The model under review builds one solid part; all positions refer to its coordinate system, in mm. A direction names the side the tool comes from. Round coordinates to 2 decimals unless told otherwise and drop trailing zeros. Write each loop counter-clockwise with the first axis right and the second up, starting at its lowest first coordinate (ties: lowest second). Pieces come first, ordered by that corner, then holes. Notation, with made-up numbers: (40.5, -35) -> (84.5, -35) arc R15 ccw to (84.5, -15) -> close; hole circle Ø5 at (70, -15.75). An arc over 180 degrees is marked (long way). Answer in a Markdown table with one row per item. Add a question column.
```python
from build123d import *

# Parameters (mm, degrees)
BOX005_W                    = 10
BOX005_H                    = 13
BOX005_DEPTH                = 4
BOX004_W                    = 3
BOX004_H                    = 31
BOX004_DEPTH                = 14
BOX003_W                    = 2
BOX003_H                    = 33
BOX003_DEPTH                = 11.2
BOX002_W                    = 9
BOX002_H                    = 35
BOX002_DEPTH                = 26
EXTRUDE_DEPTH               = 5
EXTRUDE001_DEPTH            = 5
THICKNESS_T                 = 1
BOX_W                       = 12
BOX_H                       = 31
BOX_DEPTH                   = 15
BOX001_W                    = 13
BOX001_H                    = 34
BOX001_DEPTH                = 14
CYLINDER001_W               = 48
CYLINDER001_H               = 15
CYLINDER001_ANGLE           = 60
CYLINDER001_PLACEMENT_ANGLE = 60
CYLINDER_W                  = 51
CYLINDER_H                  = 15
CYLINDER_ANGLE              = 60
CYLINDER_PLACEMENT_ANGLE    = 60


with BuildPart() as servo_wall_cutaway:
    # Box005 → Box005 (new body)
    with BuildSketch(Plane(origin=(-6, 19.5, 10), x_dir=(1, 0, 0), z_dir=(0, 0, 1))):
        with Locations((5, 6.5)):
            Rectangle(BOX005_W, BOX005_H)
    extrude(amount=BOX005_DEPTH)


with BuildPart() as slot_wall_cutout2:
    # Box004 → Box004 (new body)
    with BuildSketch(Plane(origin=(-1, 7, 14), x_dir=(1, 0, 0), z_dir=(0, 0, 1))):
        with Locations((1.5, 15.5)):
            Rectangle(BOX004_W, BOX004_H)
    extrude(amount=BOX004_DEPTH)


with BuildPart() as slot_wall_cutout1:
    # Box003 → Box003 (new body)
    with BuildSketch(Plane(origin=(-0.5, 6, 20), x_dir=(1, 0, 0), z_dir=(0, 0, 1))):
        with Locations((1, 16.5)):
            Rectangle(BOX003_W, BOX003_H)
    extrude(amount=BOX003_DEPTH)


with BuildPart() as wall_slot_finished:
    # Box002 → Box002 (new body)
    with BuildSketch(Plane(origin=(-3, 5, 0), x_dir=(1, 0, 0), z_dir=(0, 0, 1))):
        with Locations((4.5, 17.5)):
            Rectangle(BOX002_W, BOX002_H)
    extrude(amount=BOX002_DEPTH)

    # Cut003: cut slot wall cutout1
    add(slot_wall_cutout1.part, mode=Mode.SUBTRACT)

    # Cut004: cut slot wall cutout2
    add(slot_wall_cutout2.part, mode=Mode.SUBTRACT)


with BuildPart() as wall_slot_finished_1:
    # Cut004 placement: moved
    add(wall_slot_finished.part.moved(Location((-3.3, -4.4, 0))))


with BuildPart() as extrude_body:
    with BuildSketch(Plane(origin=(8.5, 45, 6), x_dir=(1, 0, 0), z_dir=(0, 1, 0))):
        with BuildLine():
            Line((5, 4), (-5, 4))
            Line((-5, 4), (-5, -3.142136))
            ThreePointArc((-5, -3.142136), (-2.53653, -3.783978), (0, -4))
            ThreePointArc((0, -4), (2.53653, -3.783978), (5, -3.142136))
            Line((5, -3.142136), (5, 4))
        make_face()
    extrude(amount=EXTRUDE_DEPTH)


with BuildPart() as extrude001:
    with BuildSketch(Plane(origin=(8.5, 45, 6), x_dir=(1, 0, 0), z_dir=(0, 1, 0))):
        with BuildLine():
            Line((5, 4), (-5, 4))
            Line((-5, 4), (-5, -3.142136))
            ThreePointArc((-5, -3.142136), (-2.53653, -3.783978), (0, -4))
            ThreePointArc((0, -4), (2.53653, -3.783978), (5, -3.142136))
            Line((5, -3.142136), (5, 4))
        make_face()
    extrude(amount=EXTRUDE001_DEPTH)


with BuildPart() as bolt_bottle_side_opening:
    # Thickness base: copy of Extrude body
    add(extrude_body.part)

    # Thickness
    thickness_openings = [bolt_bottle_side_opening.faces().sort_by_distance(p)[0] for p in [
        (8.5, 50, 5.862901),
    ]]
    offset(amount=THICKNESS_T, openings=thickness_openings)

    # Fusion: union Extrude body, Extrude001
    add(extrude_body.part)
    add(extrude001.part)


with BuildPart() as bolt_bottle_side_opening_1:
    # Fusion placement: moved
    add(bolt_bottle_side_opening.part.moved(Location((0, -7, 1))))


with BuildPart() as pullbay:
    # Box → Box (new body)
    with BuildSketch(Plane(origin=(2.5, 7, 2), x_dir=(1, 0, 0), z_dir=(0, 0, 1))):
        with Locations((6, 15.5)):
            Rectangle(BOX_W, BOX_H)
    extrude(amount=BOX_DEPTH)


with BuildPart() as cut_bay_from_case:
    # Box001 → Box001 (new body)
    with BuildSketch(Plane(origin=(2, 6, 0), x_dir=(1, 0, 0), z_dir=(0, 0, 1))):
        with Locations((6.5, 17)):
            Rectangle(BOX001_W, BOX001_H)
    extrude(amount=BOX001_DEPTH)

    # Cut001: cut pullBay
    add(pullbay.part, mode=Mode.SUBTRACT)


with BuildPart() as bottle_wall001:
    # Cylinder001 → Cylinder001 (revolve)
    with BuildSketch(Plane.XZ):
        with Locations((24, 7.5)):
            Rectangle(CYLINDER001_W, CYLINDER001_H)
    revolve(axis=Axis((0, 0, 0), (0, 0, 1)), revolution_arc=CYLINDER001_ANGLE)


with BuildPart() as bottle_wall001_1:
    # Cylinder001 placement: moved
    add(bottle_wall001.part.moved(Location((8.5, -7, 0))).rotate(Axis((8.5, -7, 0), (0, 0, 1)), CYLINDER001_PLACEMENT_ANGLE))


with BuildPart() as cut005:
    # Cylinder → Cylinder (revolve)
    with BuildSketch(Plane.XZ):
        with Locations((25.5, 7.5)):
            Rectangle(CYLINDER_W, CYLINDER_H)
    revolve(axis=Axis((0, 0, 0), (0, 0, 1)), revolution_arc=CYLINDER_ANGLE)


with BuildPart() as cut005_1:
    # Cylinder placement: moved
    add(cut005.part.moved(Location((8.5, -7, 0))).rotate(Axis((8.5, -7, 0), (0, 0, 1)), CYLINDER_PLACEMENT_ANGLE))

    # Cut: cut bottle_wall001
    add(bottle_wall001_1.part, mode=Mode.SUBTRACT)


with BuildPart() as cut005_2:
    # Cut placement: moved
    add(cut005_1.part.moved(Location((0, -2, 0))))

    # Fusion001: union cut bay from case
    add(cut_bay_from_case.part)

    # Cut002: cut bolt_bottle_side_opening
    add(bolt_bottle_side_opening_1.part, mode=Mode.SUBTRACT)

    # Fusion002: union wall slot finished
    add(wall_slot_finished_1.part)

    # Cut005: cut servo wall cutaway
    add(servo_wall_cutaway.part, mode=Mode.SUBTRACT)


solid = cut005_2.part
```
1. Add section D-D on y = 14. Write out the cut boundary in (x, z), plus the area to 3 significant figures.
2. Insertion check: pin 1 Ø12 at (x, z) = (-2.5, 9.5) entering from +Y; pin 2 Ø8 at (x, y) = (10, 25.5) entering from +Z; pin 3 Ø4 at (x, z) = (8, 15.5) entering from -Y. Each pin has a flat end and moves straight along its axis. Give the tip position at first contact, or say it passes through.
3. Add section C-C on z = 7.75. Write out the cut boundary in (x, y), plus the area to 3 significant figures.
4. Add section A-A on y = 28. Write out the cut boundary in (x, z).
5. Tool access review of faces 4 (the flat face through (2, 37, 7)), 5 (the flat face through (-1.3, 18, 20)), 6 (the flat face through (-2, 0.6, 13)), 7 (the flat face through (2.5, 38, 8)): name each direction out of +Z, -Z, +X, -X, +Y, -Y from which nothing blocks a thin tool from reaching the whole face with its end or side.
6. Mouldability with a two-part tool opening along Z and no side actions: class faces 1 (the flat face through (14.7, 23.8, 14)), 2 (the flat face through (-6, 26, 12)), 3 (the flat face through (-4.3, 18, 20)) as pulls with the +Z half, pulls with the -Z half, needs draft (parallel to the pull), parting line crosses it, or undercut.
7. Add section B-B on x = -3. Write out the cut boundary in (y, z), plus the area to 3 significant figures.
8. For L1, parallel to Y at x = -4, z = 22; L2, parallel to X at y = 27, z = 10.75; L3, parallel to X at y = 7.5, z = 8.5, list the stretches that pass through material, from the lowest coordinate up.
Filled in:
| question | item | result |
|---|---|---|
| 1 | outline | (-6.3, 0) -> (15, 0) -> (15, 14) -> (14.5, 14) -> (14.5, 2) -> (2.7, 2) -> (2.7, 26) -> (-1.3, 26) -> (-1.3, 14) -> (-4.3, 14) -> (-4.3, 26) -> (-6.3, 26) -> close |
| 1 | area | 229 mm² |
| 2 | pin 1 | y = 41.73 |
| 2 | pin 2 | z = 2 |
| 2 | pin 3 | y = 6 |
| 3 | outline | (-17, 35.17) -> (-15.5, 32.57) arc R48 cw to (2, 38.56) -> (2, 35.6) -> (-6.3, 35.6) -> (-6.3, 0.6) -> (2.7, 0.6) -> (2.7, 6) -> (15, 6) -> (15, 38.56) arc R48 cw to (32.5, 32.57) -> (34, 35.17) arc R51 ccw to (14.5, 41.65) -> (14.5, 7) -> (2.7, 7) -> (2.7, 35.6) -> (2.5, 35.6) -> (2.5, 41.65) arc R51 ccw to start |
| 3 | area | 464 mm² |
| 4 | outline | (-6.3, 0) -> (15, 0) -> (15, 14) -> (14.5, 14) -> (14.5, 2) -> (2.7, 2) -> (2.7, 10) -> (-6, 10) -> (-6, 14) -> (-4.3, 14) -> (-4.3, 26) -> (-6.3, 26) -> close; (-1.3, 14) -> (2.7, 14) -> (2.7, 26) -> (-1.3, 26) -> close |
| 5 | face 4 | +Z, -Z |
| 5 | face 5 | +Z |
| 5 | face 6 | +Z, -Z, +X, -X, -Y |
| 5 | face 7 | none |
| 6 | face 1 | pulls with the +Z half |
| 6 | face 2 | undercut |
| 6 | face 3 | needs draft |
| 7 | outline | (0.6, 0) -> (35.6, 0) -> (35.6, 26) -> (34.6, 26) -> (34.6, 20) -> (33.6, 20) -> (33.6, 14) -> (32.5, 14) -> (32.5, 10) -> (19.5, 10) -> (19.5, 14) -> (2.6, 14) -> (2.6, 20) -> (1.6, 20) -> (1.6, 26) -> (0.6, 26) -> close; (37.6, 0) -> (40.69, 0) -> (40.69, 15) -> (37.6, 15) -> close |
| 7 | area | 520 mm² |
| 8 | L1 | 0.6 to 2.6, 33.6 to 35.6 |
| 8 | L2 | -6.3 to -6, 14.5 to 15 |
| 8 | L3 | -6.3 to 2.7, 14.5 to 15 |
